Work out the finished part from the listing and answer in its coordinate system (mm). Coordinates: 2 decimals unless noted, no trailing zeros. Loops run counter-clockwise (first coordinate to the right, second up) from the corner with the lowest first, then second, coordinate; pieces in that order, holes last. Notation, with made-up numbers: (-23.75, 1) - (-1.75, 1) arc R20 cw to (-1.75, 39) - close; hole circle Ø9 at (-30.5, 74). An arc over 180 degrees is marked (long way). Write each question's results on one line, items separated by ' | '. Start each with the question number.
1. This flat-tipped pin is pushed along its axis until it touches: P1, Ø4, axis at x = -43.18, z = -25.4, coming from the +Y side. Where does it stop, or does it pass through?
2. A cutting plane is placed at D-D on y = 2.25. State how many separate pieces and enclosed holes the cut face has, then the cut area to 3 significant figures.
3. Determine the mould class of faces 1 (the flat face through (-13, 12.7, -1)), 2 (the cylindrical face through (19.5, 6.26, 12.94)), 3 (the flat face through (-1, 6, -38.1)) for opening direction Z: released by +Z, released by -Z, zero draft, split by the parting line, or undercut.
4. A cutting plane is placed at B-B on x = 0. Determine the outline of the cut face in (y, z), then the cut area to 3 significant figures.
5. A cutting plane is placed at A-A on z = -25.4. Determine the outline of the cut face in (x, y) (3 decimals).
6. A cutting plane is placed at C-C on x = -43.18. Determine the outline of the cut face in (y, z) (3 decimals).
7. Find the intervals of material crossed by line 1 along X through (y, z) = (8.75, 25.4) (3 decimals); line 2 along Z through (x, y) = (43.18, 5) (3 decimals); line 3 along Z through (x, y) = (4.5, 12.25), in increasing order. Write a range as [from, to].
from build123d import *

# Parameters (mm, degrees)
SKETCH1_W           = 111.76
SKETCH1_H           = 76.2
SKETCH1_R           = 9.68375
SKETCH1_R_2         = 2.0193
SKETCH1_R_3         = 3.175
BOSS_EXTRUDE1_DEPTH = 12.7


with BuildPart() as part:
    # Sketch1 → Boss-Extrude1 (new body)
    with BuildSketch(Plane(origin=(0, 0, 0), x_dir=(1, 0, 0), z_dir=(0, 1, 0))):
        Rectangle(SKETCH1_W, SKETCH1_H)
        Circle(SKETCH1_R, mode=Mode.SUBTRACT)
        with Locations((-20.986174507, 14.308755346)):
            Circle(SKETCH1_R_2, mode=Mode.SUBTRACT)
        with Locations((20.986174507, -14.308755346)):
            Circle(SKETCH1_R_2, mode=Mode.SUBTRACT)
        with Locations((-43.18, 25.4)):
            Circle(SKETCH1_R_3, mode=Mode.SUBTRACT)
        with Locations((-43.18, -25.4)):
            Circle(SKETCH1_R_3, mode=Mode.SUBTRACT)
        with Locations((43.18, -25.4)):
            Circle(SKETCH1_R_3, mode=Mode.SUBTRACT)
        with Locations((43.18, 25.4)):
            Circle(SKETCH1_R_3, mode=Mode.SUBTRACT)
    extrude(amount=BOSS_EXTRUDE1_DEPTH)


solid = part.part
Values:
1) P1: through
2) separate pieces: 1 | enclosed holes: 7 | area: 8,070 mm^2
3) face 1: zero draft | face 2: undercut | face 3: released by -Z
4) outline: (0, -38.1) - (12.7, -38.1) - (12.7, -9.68) - (0, -9.68) - close; (0, 9.68) - (12.7, 9.68) - (12.7, 38.1) - (0, 38.1) - close | area: 722 mm^2
5) outline: (-55.88, 0) - (-46.355, 0) - (-46.355, 12.7) - (-55.88, 12.7) - close; (-40.005, 0) - (40.005, 0) - (40.005, 12.7) - (-40.005, 12.7) - close; (46.355, 0) - (55.88, 0) - (55.88, 12.7) - (46.355, 12.7) - close
6) outline: (0, -38.1) - (12.7, -38.1) - (12.7, -28.575) - (0, -28.575) - close; (0, -22.225) - (12.7, -22.225) - (12.7, 22.225) - (0, 22.225) - close; (0, 28.575) - (12.7, 28.575) - (12.7, 38.1) - (0, 38.1) - close
7) line 1: [-55.88, -46.355], [-40.005, 40.005], [46.355, 55.88] | line 2: [-38.1, -28.575], [-22.225, 22.225], [28.575, 38.1] | line 3: [-38.1, -8.57], [8.57, 38.1]
